Design review of the part built by this model. Coordinates are the model's own, in mm. Face numbers are marked on the shaded views. A direction names the side the tool comes from. Coordinates: 2 decimals unless noted, no trailing zeros. Write each loop counter-clockwise with the first axis right and the second up, starting at its lowest first coordinate (ties: lowest second). Pieces come first, ordered by that corner, then holes. Notation, with made-up numbers: (-4, 64.5) - (18, 64.5) arc R23 cw to (18, 102.5) - close; hole circle Ø9 at (-2.5, -26). An arc over 180 degrees is marked (long way). One line per item, written item: value.
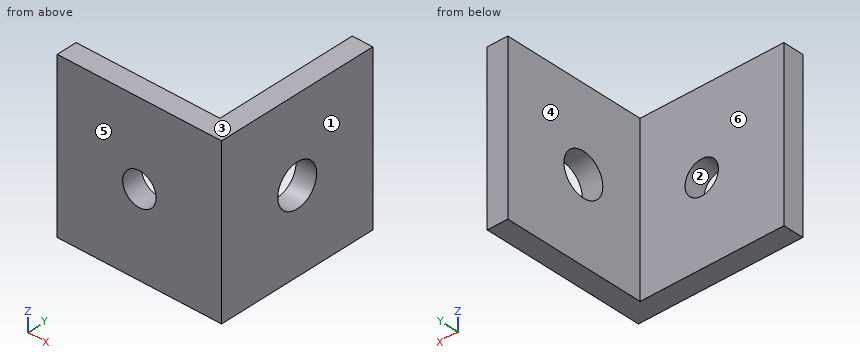
from build123d import *

# Parameters (mm, degrees)
BOSS_EXTRUDE1_DEPTH              = 25.4
F_13_64_0_20313_DIAMETER_HOLE1_D = 5.159375
F_0_257_DIAMETER_HOLE1_D         = 6.5278


with BuildPart() as part:
    # Sketch1 → Boss-Extrude1 (new body)
    with BuildSketch(Plane.XY):
        Polygon((0, 3.175), (22.225, 3.175), (22.225, 25.4), (25.4, 25.4), (25.4, 0), (0, 0), align=None)
    extrude(amount=BOSS_EXTRUDE1_DEPTH)

    # 13/64 (0.20313) Diameter Hole1 (through all)
    with Locations(Plane(origin=(0, 0, 0), x_dir=(-1, 0, 0), z_dir=(0, -1, 0))):
        with Locations((-12.7, -12.7)):
            Hole(F_13_64_0_20313_DIAMETER_HOLE1_D / 2)

    # F (0.257) Diameter Hole1 (through all)
    with Locations(Plane(origin=(25.4, 0, 0), x_dir=(0, 0, -1), z_dir=(1, 0, 0))):
        with Locations((-12.7, 12.7)):
            Hole(F_0_257_DIAMETER_HOLE1_D / 2)


solid = part.part
1. Insertion check: pin 1 Ø3 at (x, z) = (12.7, 12.7) entering from -Y; pin 2 Ø2 at (x, z) = (14.5, 15) entering from +Y (3 decimals). Each pin has a flat end and moves straight along its axis. Give the tip position at first contact, or say it passes through.
Answer block:
pin 1: passes through
pin 2: stops at y = 3.175
2. Wall thickness on line 1 along X through (y, z) = (5.75, 3) (3 decimals); line 2 along Y through (x, z) = (1.5, 11) (3 decimals); line 3 along Z through (x, y) = (12.7, 2.4): over which ranges is each line inside the solid? List them lowest first.
Answer block:
line 1: x = 22.225 to 25.4
line 2: y = 0 to 3.175
line 3: z = 0 to 10.12, 15.28 to 25.4
3. For the marked faces 5 and 6, list the 3-axis set-ups (+Z, -Z, +X, -X, +Y, -Y) from which the entire face can be reached by the end or side of a thin tool; tool diameter is ignored.
Answer block:
face 5: +Z, -Z, +X, -X, -Y
face 6: +Z, -Z, -X, +Y
4. Consider section B-B, the plane z = 12.7. Write out the cut boundary in (x, y) (3 decimals).
Answer block:
outline: (0, 0) - (10.12, 0) - (10.12, 3.175) - (0, 3.175) - close; (15.28, 0) - (25.4, 0) - (25.4, 9.436) - (22.225, 9.436) - (22.225, 3.175) - (15.28, 3.175) - close; (22.225, 15.964) - (25.4, 15.964) - (25.4, 25.4) - (22.225, 25.4) - close
5. Consider section A-A, the plane y = 12.7. Write out the cut boundary in (x, z) (3 decimals), then the cut area to 3 significant figures.
Answer block:
outline: (22.225, 0) - (25.4, 0) - (25.4, 9.436) - (22.225, 9.436) - close; (22.225, 15.964) - (25.4, 15.964) - (25.4, 25.4) - (22.225, 25.4) - close
area: 59.9 mm^2
6. Consider section D-D, the plane x = 22.75. Write out the cut boundary in (y, z).
Answer block:
outline: (0, 0) - (25.4, 0) - (25.4, 25.4) - (0, 25.4) - close; hole circle Ø6.53 at (12.7, 12.7)
7. Mouldability with a two-part tool opening along X and no side actions: class the marked faces 1, 2, 3 and 4 as released by +X, released by -X, zero draft, split by the parting line, or undercut.
Answer block:
face 1: released by +X
face 2: undercut
face 3: zero draft
face 4: released by -X
8. Consider section C-C, the plane x = 12.7. Write out the cut boundary in (y, z) (3 decimals), then the cut area to 3 significant figures.
Answer block:
outline: (0, 0) - (3.175, 0) - (3.175, 10.12) - (0, 10.12) - close; (0, 15.28) - (3.175, 15.28) - (3.175, 25.4) - (0, 25.4) - close
area: 64.3 mm^2
